Geometry check sheet. Reference: the model listing, model coordinates, mm. Round coordinates to 2 decimals unless told otherwise and drop trailing zeros. Order: outer loops, then holes, each group sorted by start corner. A loop starts at its lowest first (then second) coordinate and runs counter-clockwise, first axis right, second up. Notation, with made-up numbers: (8.5, -5) - (56.5, -5) arc R24 cw to (56.5, 21) - close; hole circle Ø3 at (31, 71). An arc over 180 degrees is marked (long way). Return JSON: item names as keys, results as strings. Group by question number.
Q1. Sectioned sample at A-A, the plane z = -19. Record the cut outline in (x, y).
Q2. Material ranges on line 1 along Y through (x, z) = (-11.5, 12); line 2 along X through (y, z) = (18.75, -7); line 3 along Z through (x, y) = (1, 19), recorded low to high.
Q3. Gauge pin test, flat ends, axial feed: pin 1 Ø15 at (x, z) = (10, 6.5) entering from +Y; pin 2 Ø8 at (x, z) = (18, 16.5) entering from +Y; pin 3 Ø2 at (y, z) = (18.5, -6.5) entering from +X; pin 4 Ø3 at (y, z) = (18.5, 3.5) entering from -X. Record the tip position at first contact, or that the pin passes through.
Q4. Sectioned sample at B-B, the plane x = 0. Record the cut outline in (y, z), then the cut area to 3 significant figures.
Q5. Sectioned sample at D-D, the plane z = 0. Record the cut outline in (x, y).
Q6. Sectioned sample at C-C, the plane x = -19. Record the cut outline in (y, z), then the cut area to 3 significant figures.
Q7. Draft check along X on faces 1 (the cylindrical face through (-17.99, 3.04, 17.89)), 2 (the cylindrical face through (-9.76, 15.89, -2.17)), 3 (the flat face through (25, 4, 0)), 4 (the flat face through (11, 8, 0)). Enter one of: pulls with the +X half, pulls with the -X half, needs draft (parallel to the pull), parting line crosses it, or undercut.
```python
from build123d import *

# Parameters (mm, degrees)
SKETCH1_W                    = 50
SKETCH1_H                    = 50
BOSS_EXTRUDE1_DEPTH          = 8
SKETCH2_R                    = 10
BOSS_EXTRUDE2_DEPTH          = 16
SKETCH3_R                    = 1.5
CUT_EXTRUDE1_DEPTH           = 8
CHAMFER1_SIZE                = 2
CIRPATTERN3_COUNT            = 4
CHAMFER1_OF_CIRPATTERN3_SIZE = 2


with BuildPart() as part:
    # Sketch1 → Boss-Extrude1 (new body)
    with BuildSketch(Plane(origin=(0, 0, 0), x_dir=(1, 0, 0), z_dir=(0, 1, 0))):
        Rectangle(SKETCH1_W, SKETCH1_H)
    extrude(amount=BOSS_EXTRUDE1_DEPTH)

    # Sketch2 → Boss-Extrude2 (add)
    with BuildSketch(Plane(origin=(0, 8, 0), x_dir=(1, 0, 0), z_dir=(0, 1, 0))):
        with Locations(Location((0, 0, 0), (0, 0, 270))):
            Circle(SKETCH2_R)
    extrude(amount=BOSS_EXTRUDE2_DEPTH)

    # Sketch3 → Cut-Extrude1 (cut)
    with BuildSketch(Plane(origin=(0, 8, 0), x_dir=(1, 0, 0), z_dir=(0, 1, 0))):
        with Locations(Location((-19, -19, 0), (0, 0, 270))):
            Circle(SKETCH3_R)
    cut_extrude1 = extrude(amount=-CUT_EXTRUDE1_DEPTH, mode=Mode.SUBTRACT)

    # Chamfer1
    chamfer1_edges = [part.edges().sort_by_distance(p)[0] for p in [
        (-19, 8, 17.5),
    ]]
    chamfer(chamfer1_edges, length=CHAMFER1_SIZE)

    # CirPattern3: Cut-Extrude1 ×4 about axis
    cirpattern3_axis = Axis((0, 0, 0), (0, 1, 0))
    for i in range(1, CIRPATTERN3_COUNT):
        add(cut_extrude1.rotate(cirpattern3_axis, i * 360 / CIRPATTERN3_COUNT), mode=Mode.SUBTRACT)

    # Chamfer1 of CirPattern3
    chamfer1_of_cirpattern3_edges = [part.edges().sort_by_distance(p)[0] for p in [
        (17.5, 8, 19),
        (19, 8, -17.5),
        (-17.5, 8, -19),
    ]]
    chamfer(chamfer1_of_cirpattern3_edges, length=CHAMFER1_OF_CIRPATTERN3_SIZE)


solid = part.part
```
Reply:
{
 "1": {"outline": "(-25, 0) - (-20.5, 0) - (-20.5, 6) - (-22.5, 8) - (-25, 8) - close; (-17.5, 0) - (17.5, 0) - (17.5, 6) - (15.5, 8) - (-15.5, 8) - (-17.5, 6) - close; (20.5, 0) - (25, 0) - (25, 8) - (22.5, 8) - (20.5, 6) - close"},
 "2": {"line 1": "0 to 8", "line 2": "-7.14 to 7.14", "line 3": "-9.95 to 9.95"},
 "3": {"pin 1": "y = 24", "pin 2": "y = 8", "pin 3": "x = 8.35", "pin 4": "x = -9.8"},
 "4": {"outline": "(0, -25) - (8, -25) - (8, -10) - (24, -10) - (24, 10) - (8, 10) - (8, 25) - (0, 25) - close", "area": "720 mm^2"},
 "5": {"outline": "(-25, 0) - (25, 0) - (25, 8) - (10, 8) - (10, 24) - (-10, 24) - (-10, 8) - (-25, 8) - close"},
 "6": {"outline": "(0, -25) - (8, -25) - (8, -22.5) - (6, -20.5) - (0, -20.5) - close; (0, -17.5) - (6, -17.5) - (8, -15.5) - (8, 15.5) - (6, 17.5) - (0, 17.5) - close; (0, 20.5) - (6, 20.5) - (8, 22.5) - (8, 25) - (0, 25) - close", "area": "344 mm^2"},
 "7": {"face 1": "undercut", "face 2": "parting line crosses it", "face 3": "pulls with the +X half", "face 4": "needs draft"}
}
